Job drawing, mm, ordinate dimensions from the low corner. One solid piece. A direction names the side the tool comes from. Round coordinates to 2 decimals unless told otherwise and drop trailing zeros. Loops run counter-clockwise (first coordinate to the right, second up) from the corner with the lowest first, then second, coordinate; pieces in that order, holes last.
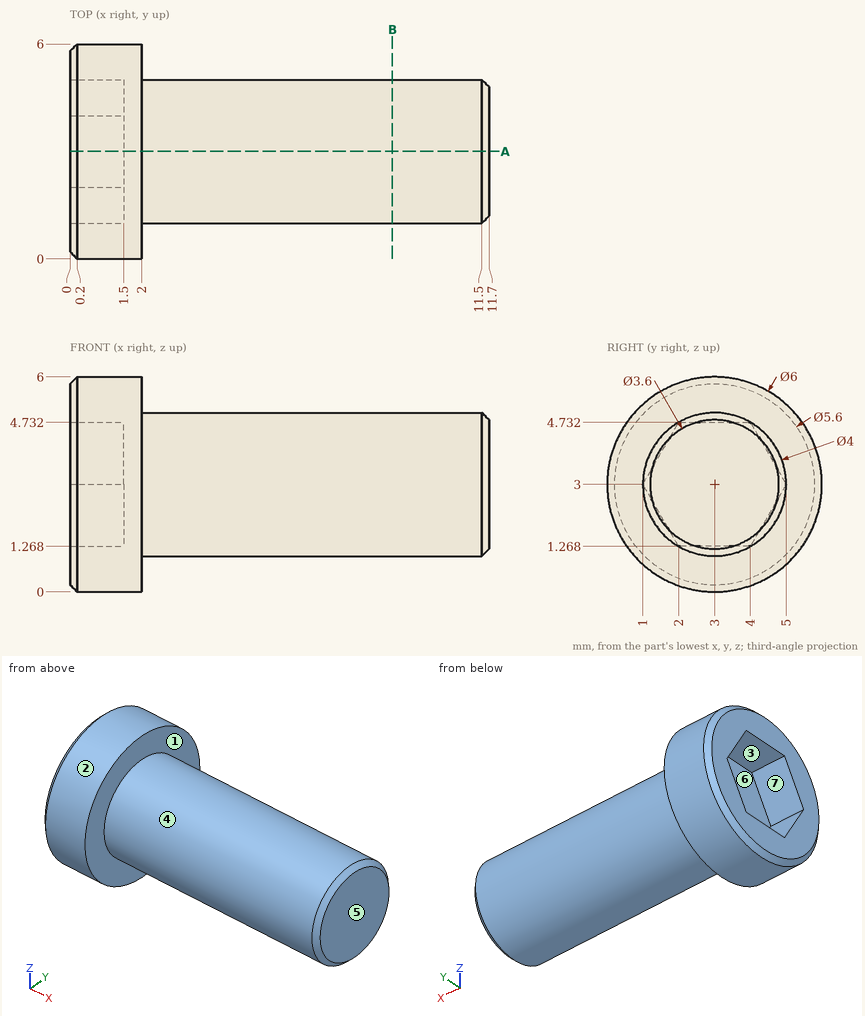
Item 1: Cut at A-A, the plane y = 3. Give the cut face in (x, z), plus the area to 3 significant figures.
Answers follow:
outline: (0, 0.2) - (0.2, 0) - (2, 0) - (2, 1) - (11.5, 1) - (11.7, 1.2) - (11.7, 4.8) - (11.5, 5) - (2, 5) - (2, 6) - (0.2, 6) - (0, 5.8) - (0, 4.73) - (1.5, 4.73) - (1.5, 1.27) - (0, 1.27) - close
area: 45.5 mm2
Item 2: Cut at B-B, the plane x = 9. Give the cut face in (y, z), plus the area to 3 significant figures.
Answers follow:
outline: circle Ø4 at (3, 3)
area: 12.6 mm2
Item 3: Flat gauge pins, fed straight in: P1, Ø1.7, axis at y = 2.5, z = 4, coming from the -X side; P2, Ø3, axis at x = 3, z = 1.5, coming from the -Y side; P3, Ø1, axis at x = 3, z = 1.5, coming from the +Y side; P4, Ø1.5, axis at x = 3, y = 3, coming from the +Z side. Where does each tip first touch, or does it go through?
Answers follow:
P1: stops at x = 0
P2: stops at y = 0.02
P3: stops at y = 4.73
P4: stops at z = 5
Item 4: Two-plate mould, pull along Y, no slides. Class the marked faces 4, 5, 6 and 7: released by +Y, released by -Y, zero draft, split by the parting line, or undercut.
Answers follow:
face 4: split by the parting line
face 5: zero draft
face 6: undercut
face 7: undercut
Item 5: Probe line 1 (X direction, y = 4.25, z = 3.6); line 2 (X direction, y = 5.05, z = 3.7); line 3 (Y direction, x = 1, z = 4.1) (3 decimals). List the from-to ranges inside material, lowest first.
Answers follow:
line 1: x = 1.5 to 11.7
line 2: x = 0 to 2
line 3: y = 0.209 to 1.635, 4.365 to 5.791
Item 6: 3-axis set-ups, long thin cutter, end or side, ignore diameter. For the marked faces 1, 2 and 3: which of +Z, -Z, +X, -X, +Y, -Y reach the whole face in a straight line?
Answers follow:
face 1: +X
face 2: +X, -X
face 3: -X
